from build123d import *

# Parameters (mm, degrees)
BOSS_EXTRUDE1_DEPTH              = 5
SLOT_DEPTH                       = 11
F_10_5_10_5_DIAMETER_HOLE1_D     = 10.5
F_10_5_10_5_DIAMETER_HOLE1_DEPTH = 15
F_10_5_10_5_DIAMETER_HOLE1_TIP   = 3.15451825
CBORE_FOR_M5_SHCS2_D             = 5.5
CBORE_FOR_M5_SHCS2_DEPTH         = 21.6
CBORE_FOR_M5_SHCS2_CBORE_D       = 10
CBORE_FOR_M5_SHCS2_CBORE_DEPTH   = 5
CBORE_FOR_M5_SHCS2_TIP           = 1.652366702
CUT_EXTRUDE3_DEPTH               = 11
FILLET1_R                        = 10
CHAMFER1_SIZE                    = 1


with BuildPart() as part:
    # Sketch1 → Boss-Extrude1 (new body, symmetric)
    with BuildSketch(Plane(origin=(0, 0, 0), x_dir=(1, 0, 0), z_dir=(0, 1, 0))):
        with BuildLine():
            Line((-390, 90), (34.468189123, 90))
            Line((34.468189123, 90), (9.659258263, -2.588190451))
            ThreePointArc((9.659258263, -2.588190451), (5.03987296, -8.63711066), (-2.499017827, -9.682711908))
            Line((-2.499017827, -9.682711908), (-20, -5.16587129))
            Line((-20, -5.16587129), (-60, 29.405996647))
            Line((-60, 29.405996647), (-391.218693434, 70.074538484))
            ThreePointArc((-391.218693434, 70.074538484), (-399.981347984, 80.610485395), (-390, 90))
        make_face()
    extrude(amount=BOSS_EXTRUDE1_DEPTH, both=True)

    # Sketch4 → Slot (cut, through all)
    with BuildSketch(Plane(origin=(0, 5, 0), x_dir=(1, 0, 0), z_dir=(0, 1, 0))):
        with BuildLine():
            Line((-30, 26.591016), (0, 26.591016))
            ThreePointArc((0, 26.591016), (8.05, 34.641016), (0, 42.691016))
            Line((0, 42.691016), (-30, 42.691016))
            ThreePointArc((-30, 42.691016), (-43.362313367, 47.226910181), (-51.202071887, 58.95993796))
            ThreePointArc((-51.202071887, 58.95993796), (-61.061268102, 64.652147549), (-66.75347769, 54.792951334))
            ThreePointArc((-66.75347769, 54.792951334), (-53.163372374, 34.453921402), (-30, 26.591016))
        make_face()
    extrude(amount=-SLOT_DEPTH, mode=Mode.SUBTRACT)

    # Ø10.5 (10.5) Diameter Hole1
    with Locations(Plane(origin=(0, 5, 0), x_dir=(1, 0, 0), z_dir=(0, 1, 0))):
        with Locations((0, 0)):
            Hole(F_10_5_10_5_DIAMETER_HOLE1_D / 2, depth=F_10_5_10_5_DIAMETER_HOLE1_DEPTH)
            with Locations((0, 0, -(F_10_5_10_5_DIAMETER_HOLE1_DEPTH + F_10_5_10_5_DIAMETER_HOLE1_TIP / 2))):  # 118° drill point
                Cone(0, F_10_5_10_5_DIAMETER_HOLE1_D / 2, F_10_5_10_5_DIAMETER_HOLE1_TIP, mode=Mode.SUBTRACT)

    # CBORE for M5 SHCS2
    with Locations(Plane(origin=(0, -5, 0), x_dir=(-1, 0, 0), z_dir=(0, -1, 0))):
        with Locations((390, 80), (240, 80)):
            CounterBoreHole(CBORE_FOR_M5_SHCS2_D / 2, CBORE_FOR_M5_SHCS2_CBORE_D / 2, CBORE_FOR_M5_SHCS2_CBORE_DEPTH, depth=CBORE_FOR_M5_SHCS2_DEPTH)
            with Locations((0, 0, -(CBORE_FOR_M5_SHCS2_DEPTH + CBORE_FOR_M5_SHCS2_TIP / 2))):  # 118° drill point
                Cone(0, CBORE_FOR_M5_SHCS2_D / 2, CBORE_FOR_M5_SHCS2_TIP, mode=Mode.SUBTRACT)

    # Sketch13 → Cut-Extrude3 (cut, through all)
    with BuildSketch(Plane(origin=(0, 5, 0), x_dir=(1, 0, 0), z_dir=(0, 1, 0))):
        Polygon((-5.531810877, 90), (34.468189123, 90), (26.42971335, 60), align=None)
    extrude(amount=-CUT_EXTRUDE3_DEPTH, mode=Mode.SUBTRACT)

    # Fillet1
    fillet1_edges = [part.edges().sort_by_distance(p)[0] for p in [
        (-20, 0, 5.16587129),
        (-60, 0, -29.405996647),
        (26.42971335, 0, -60),
        (-5.531810877, 0, -90),
    ]]
    fillet(fillet1_edges, radius=FILLET1_R)

    # Chamfer1
    chamfer1_edges = [part.edges().sort_by_distance(p)[0] for p in [
        (-399.981347984, -5, -80.610485395),
        (5.03987296, 5, 8.63711066),
        (17.26978309, 5, -25.814674877),
        (-399.981347984, 5, -80.610485395),
        (9.709435896, 5, -75.694130232),
        (9.709435896, -5, -75.694130232),
        (-199.744878532, 5, -90),
        (-39.735397279, 5, -11.891367421),
        (17.26978309, -5, -25.814674877),
        (-10.11553696, 5, 7.716959206),
        (-19.874383451, 5, 4.92614185),
        (24.83814676, 5, -59.546431893),
        (-5.80958377, 5, -89.298189314),
        (-199.744878532, -5, -90),
        (-10.11553696, -5, 7.716959206),
        (5.03987296, -5, 8.63711066),
        (-39.735397279, -5, -11.891367421),
        (-19.874383451, -5, 4.92614185),
        (24.83814676, -5, -59.546431893),
        (-5.80958377, -5, -89.298189314),
        (-60.183408772, -5, -28.992469299),
        (-227.118878147, 5, -49.925614719),
        (-60.183408772, 5, -28.992469299),
        (-227.118878147, -5, -49.925614719),
    ]]
    chamfer(chamfer1_edges, length=CHAMFER1_SIZE)


solid = part.part
Check sheet for the modelled part. Datum: model origin and axes. Units: mm. A direction names the side the tool comes from. Round coordinates to 2 decimals unless told otherwise and drop trailing zeros. Order: outer loops, then holes, each group sorted by start corner. A loop starts at its lowest first (then second) coordinate and runs counter-clockwise, first axis right, second up.
(1) Cross-section at A-A, the plane y = 2. Enter the section's corners in (x, z), and give its area (3 significant figures).
(2) Cross-section at C-C, the plane z = -21. Enter the section's corners in (x, y), and give its area (3 significant figures).
(3) Cross-section at B-B, the plane x = -167. Enter the section's corners in (y, z), and give its area (3 significant figures).
(4) Draft check along Z on faces 4 (the flat face through (-392.2, 0, -77.8)), 5 (the cylindrical face through (24.817, -0.056, -59.619)), 6 (the flat face through (-39.48, 0.06, -11.67)), 7 (the cylindrical face through (-5.86, -0.06, -89.32)). Enter one of: pulls with the +Z half, pulls with the -Z half, needs draft (parallel to the pull), parting line crosses it, or undercut.
(5) Go/stop test with flat-tipped pins: P1, Ø3, axis at x = -17.5, y = -2, coming from the +Z side; P2, Ø11, axis at x = -237.5, z = -81, coming from the -Y side; P3, Ø3, axis at x = -46, y = -1.5, coming from the +Z side; P4, Ø5, axis at y = 2.5, z = -22, coming from the -X side. Record where each tip stops, or that it passes through.
(6) Access from +Z, -Z, +X, -X, +Y, -Y to the whole of each face (thin tool, end or side, straight path). Record for faces 1 (the cylindrical face through (-394.619, -2.535, -78.085)), 2 (the flat face through (-224.821, 0.056, -49.644)), 3 (the cylindrical face through (8.048, 0.07, -34.464)).
(7) Scan lines: probe 1 along X at (y, z) = (-1.2, -80); probe 2 along X at (y, z) = (0.25, -81); probe 3 along Z at (x, y) = (-390, -3). Record each from-to range of solid material in increasing order.
Check sheet entries:
1. outline: (-391.22, -70.07) arc R10 ccw to (-390, -90) - (-9.49, -90) arc R10 ccw to (-2.65, -87.29) - (22.06, -64.1) arc R10 ccw to (24.88, -54.22) - (9.66, 2.59) arc R10 ccw to (-2.5, 9.68) - (-17.73, 5.75) arc R10 ccw to (-21.77, 3.63) - (-57.7, -27.42) arc R10 cw to (-63.02, -29.78) - close; hole circle Ø5.5 at (-390, -80); hole circle Ø5.5 at (-240, -80); hole (-66.75, -54.79) arc R8.05 ccw to (-51.2, -58.96) arc R21.95 cw to (-30, -42.69) - (0, -42.69) arc R8.05 ccw to (0, -26.59) - (-30, -26.59) arc R38.05 ccw to start; hole circle Ø10.5 at (0, 0)
1. area: 18,600 mm2
2. outline: (-50.27, -4) - (-48.74, -5) - (14.94, -5) - (15.98, -4) - (15.98, 4) - (14.94, 5) - (-48.74, 5) - (-50.27, 4) - close
2. area: 660 mm2
3. outline: (-5, -89) - (-4, -90) - (4, -90) - (5, -89) - (5, -43.55) - (4, -42.54) - (-4, -42.54) - (-5, -43.55) - close
3. area: 473 mm2
4. face 4: undercut
4. face 5: parting line crosses it
4. face 6: pulls with the +Z half
4. face 7: pulls with the -Z half
5. P1: stops at z = 6.2
5. P2: stops at y = -5
5. P3: stops at z = -16.01
5. P4: stops at x = -54.32
6. face 1: -Y
6. face 2: +Z, -X, +Y, -Y
6. face 3: +Y, -Y
7. probe 1: x = -400 to -395, -385 to -245, -235 to 5.12
7. probe 2: x = -399.95 to -392.56, -387.44 to -242.56, -237.44 to 4.06
7. probe 3: z = -90 to -85, -75 to -69.92
